from build123d import *

# Parameters (mm, degrees)
SKETCH1_R           = 19.05
BOSS_EXTRUDE1_DEPTH = 31.75
SKETCH2_R           = 3.175
CUT_EXTRUDE1_DEPTH  = 108.073506434


with BuildPart() as part:
    # Sketch1 → Boss-Extrude1 (new, symmetric)
    with BuildSketch(Plane.XY):
        with BuildLine():
            Line((-82.55, 33.3502), (-82.55, 25.4))
            Line((-82.55, 25.4), (-39.7002, 25.4))
            ThreePointArc((-39.7002, 25.4), (-30.719943879, 21.680256121), (-27.0002, 12.7))
            Line((-27.0002, 12.7), (-27.0002, 0))
            ThreePointArc((-27.0002, 0), (0, -27.0002), (27.0002, 0))
            Line((27.0002, 0), (27.0002, 12.7))
            ThreePointArc((27.0002, 12.7), (30.719943879, 21.680256121), (39.7002, 25.4))
            Line((39.7002, 25.4), (82.55, 25.4))
            Line((82.55, 25.4), (82.55, 33.3502))
            Line((82.55, 33.3502), (-82.55, 33.3502))
        make_face()
        Circle(SKETCH1_R, mode=Mode.SUBTRACT)
    extrude(amount=BOSS_EXTRUDE1_DEPTH, both=True)

    # Sketch2 → Cut-Extrude1 (cut, through all)
    with BuildSketch(Plane(origin=(0, 33.3502, 0), x_dir=(1, 0, 0), z_dir=(0, 1, 0))):
        with Locations(Location((-63.5, 15.875, 0), (0, 0, 180))):
            Circle(SKETCH2_R)
        with Locations(Location((-63.5, -15.875, 0), (0, 0, 180))):
            Circle(SKETCH2_R)
        with Locations(Location((63.5, -15.875, 0), (0, 0, 180))):
            Circle(SKETCH2_R)
        with Locations(Location((63.5, 15.875, 0), (0, 0, 180))):
            Circle(SKETCH2_R)
    extrude(amount=-CUT_EXTRUDE1_DEPTH, mode=Mode.SUBTRACT)


solid = part.part
Can you work these out from the model? Positions are in its coordinate system, mm. A direction names the side the tool comes from. Round coordinates to 2 decimals unless told otherwise and drop trailing zeros. Loops run counter-clockwise (first coordinate to the right, second up) from the corner with the lowest first, then second, coordinate; pieces in that order, holes last. Notation, with made-up numbers: (-22, -37.75) - (-18, -37.75) arc R23 cw to (-18, -22.75) - close; hole circle Ø3 at (50.25, 52). An arc over 180 degrees is marked (long way). Answer in a Markdown table with one row per item. Add a question column.
Q1. We'd pull the mould along Z, two halves only. Please class faces 4 (the cylindrical face through (-66.53, 29.43, 16.83)), 5 (the flat face through (0, 21, -31.75)), 6 (the cylindrical face through (60.47, 29.43, 16.83)), 7 (the cylindrical face through (-0.594, -26.994, 0.444)): pulls with the +Z half, pulls with the -Z half, needs draft (parallel to the pull), parting line crosses it, or undercut.
Q2. Which directions (+Z, -Z, +X, -X, +Y, -Y) give clear straight access to the entire face, cutting with the end or side of a thin tool? Please do faces 1 (the flat face through (-27, 6, 0)), 2 (the flat face through (61, 25.4, 0)), 3 (the flat face through (0, 21, 31.75)).
Q3. I want a section at A-A on x = -63.5. List the corners of the cut face in (y, z) for me.
Q4. For pin 1 Ø2 at (y, z) = (0, 24.5) entering from +X; pin 2 Ø6 at (y, z) = (16, 0) entering from -X; pin 3 Ø8.5 at (x, z) = (63.5, -15.875) entering from -Y; pin 4 Ø5 at (x, z) = (-63.5, 15.875) entering from +Y, each with a flat end and sliding along its axis, tell me the tip position at first contact or that it passes through.
Q5. I want a section at D-D on x = -33. List the corners of the cut face in (y, z) for me, and give its area (3 significant figures).
Q6. I want a section at C-C on y = -17. List the corners of the cut face in (x, z) for me.
Q7. I want a section at B-B on x = 0. List the corners of the cut face in (y, z) for me, and give its area (3 significant figures).
Q8. I need wall thicknesses on L1, parallel to Z at x = 63.5, y = 28; L2, parallel to Y at x = -39.5, z = -24.5; L3, parallel to X at y = -15, z = -18. Which ranges of each line are inside material? Lowest first, please.
A:
| question | item | result |
|---|---|---|
| 1 | face 4 | undercut |
| 1 | face 5 | pulls with the -Z half |
| 1 | face 6 | undercut |
| 1 | face 7 | needs draft |
| 2 | face 1 | +Z, -Z, -X, -Y |
| 2 | face 2 | +Z, -Z, +X, -Y |
| 2 | face 3 | +Z, +X, -X, +Y, -Y |
| 3 | outline | (25.4, -31.75) - (33.35, -31.75) - (33.35, -19.05) - (25.4, -19.05) - close; (25.4, -12.7) - (33.35, -12.7) - (33.35, 12.7) - (25.4, 12.7) - close; (25.4, 19.05) - (33.35, 19.05) - (33.35, 31.75) - (25.4, 31.75) - close |
| 4 | pin 1 | x = 27 |
| 4 | pin 2 | x = -28.67 |
| 4 | pin 3 | y = 25.4 |
| 4 | pin 4 | through |
| 5 | outline | (23.49, -31.75) - (33.35, -31.75) - (33.35, 31.75) - (23.49, 31.75) - close |
| 5 | area | 626 mm^2 |
| 6 | outline | (-20.98, -31.75) - (-8.6, -31.75) - (-8.6, 31.75) - (-20.98, 31.75) - close; (8.6, -31.75) - (20.98, -31.75) - (20.98, 31.75) - (8.6, 31.75) - close |
| 7 | outline | (-27, -31.75) - (-19.05, -31.75) - (-19.05, 31.75) - (-27, 31.75) - close; (19.05, -31.75) - (33.35, -31.75) - (33.35, 31.75) - (19.05, 31.75) - close |
| 7 | area | 1,410 mm^2 |
| 8 | L1 | -31.75 to -19.05, -12.7 to 12.7, 19.05 to 31.75 |
| 8 | L2 | 25.4 to 33.35 |
| 8 | L3 | -22.45 to -11.74, 11.74 to 22.45 |
